Source: CAD feature listing. Evaluate the final solid. Frame: model axes, mm. Round coordinates to 2 decimals unless told otherwise and drop trailing zeros. Order: outer loops, then holes, each group sorted by start corner. A loop starts at its lowest first (then second) coordinate and runs counter-clockwise, first axis right, second up. Notation, with made-up numbers: (-3.5, -12.75) - (9.5, -12.75) arc R22 cw to (9.5, 14.25) - close; hole circle Ø10 at (6, -13). An arc over 180 degrees is marked (long way). Return JSON: item names as keys, results as strings. Group by question number.
1) Section C-C, the plane y = -52.5. Return loops of the section in (x, z).
2) Section B-B, the plane y = -175. Return loops of the section in (x, z), plus the area to 3 significant figures.
3) Section A-A, the plane x = 0. Return loops of the section in (y, z) (3 decimals), plus the area to 3 significant figures.
4) Ray query, line 1 (Y direction, x = 0.25, z = 5.75); line 2 (X direction, y = -215, z = 1.75) (3 decimals); line 3 (Y direction, x = 2, z = 5.5). Return the intervals inside material, ascending. Write a range as from..to.
5) Contact query for flat-ended pins moving along their axis: P1, Ø5, axis at x = 0, y = -175, coming from the +Z side; P2, Ø0.5, axis at y = -136.5, z = 4.5, coming from the -X side. Output: stop coordinate, or through.
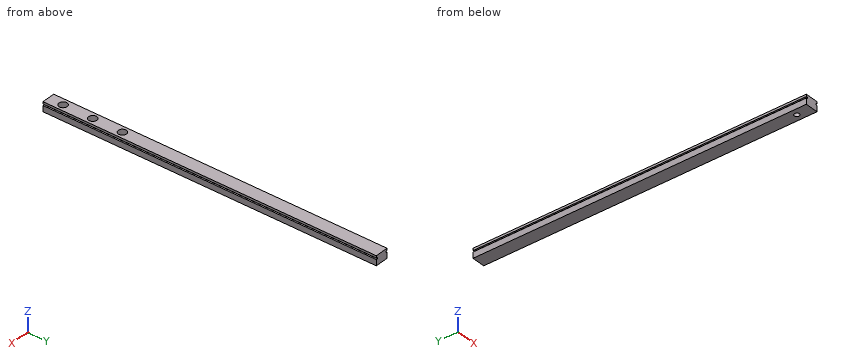
```python
from build123d import *

# Parameters (mm, degrees)
F1_DEPTH = 225
F2_R     = 2.75
F3_DEPTH = 4.25
F4_R     = 1.675
F5_DEPTH = 2.201


with BuildPart() as f1:
    # F0 (on Front) → F1 (new body)
    with BuildSketch(Plane.XZ):
        Polygon((-4.45, 4), (-4.45, 0), (4.45, 0), (4.45, 4), (3.45, 4), (3.45, 4.95), (4.45, 4.95), (4.45, 6.45), (-4.45, 6.45), (-4.45, 4.95), (-3.45, 4.95), (-3.45, 4), align=None)
    extrude(amount=F1_DEPTH)

    # F2 (on face) → F3 (cut)
    with BuildSketch(Plane.XY.offset(6.45)):
        with Locations((0, -215)):
            Circle(F2_R)
        with Locations((0, -195)):
            Circle(F2_R)
        with Locations((0, -175)):
            Circle(F2_R)
    extrude(amount=-F3_DEPTH, mode=Mode.SUBTRACT)

    # F4 (on face) → F5 (cut, through all)
    with BuildSketch(Plane.XY.offset(2.2)):
        with Locations((0, -215)):
            Circle(F4_R)
    extrude(amount=-F5_DEPTH, mode=Mode.SUBTRACT)


solid = f1.part
```
Geometry check:
{
 "1": {"outline": "(-4.45, 0) - (4.45, 0) - (4.45, 4) - (3.45, 4) - (3.45, 4.95) - (4.45, 4.95) - (4.45, 6.45) - (-4.45, 6.45) - (-4.45, 4.95) - (-3.45, 4.95) - (-3.45, 4) - (-4.45, 4) - close"},
 "2": {"outline": "(-4.45, 0) - (4.45, 0) - (4.45, 4) - (3.45, 4) - (3.45, 4.95) - (4.45, 4.95) - (4.45, 6.45) - (2.75, 6.45) - (2.75, 2.2) - (-2.75, 2.2) - (-2.75, 6.45) - (-4.45, 6.45) - (-4.45, 4.95) - (-3.45, 4.95) - (-3.45, 4) - (-4.45, 4) - close", "area": "32.1 mm2"},
 "3": {"outline": "(-225, 0) - (-216.675, 0) - (-216.675, 2.2) - (-217.75, 2.2) - (-217.75, 6.45) - (-225, 6.45) - close; (-213.325, 0) - (0, 0) - (0, 6.45) - (-172.25, 6.45) - (-172.25, 2.2) - (-177.75, 2.2) - (-177.75, 6.45) - (-192.25, 6.45) - (-192.25, 2.2) - (-197.75, 2.2) - (-197.75, 6.45) - (-212.25, 6.45) - (-212.25, 2.2) - (-213.325, 2.2) - close", "area": "1,370 mm2"},
 "4": {"line 1": "-225..-217.74, -212.26..-197.74, -192.26..-177.74, -172.26..0", "line 2": "-4.45..-1.675, 1.675..4.45", "line 3": "-225..-216.89, -213.11..-196.89, -193.11..-176.89, -173.11..0"},
 "5": {"P1": "z = 2.2", "P2": "x = -3.45"}
}
